```python
from build123d import *

# Parameters (mm, degrees)
Y_KSEKLIK_EKSTR_ZYON2_DEPTH       = 14
KES_EKSTR_ZYON1_REACH             = 47.202
IZIM2_R                           = 2.85
KES_EKSTR_ZYON1_DIRECTION_2_DEPTH = 46.202322949


with BuildPart() as part:
    # Çizim1 → Yükseklik-Ekstrüzyon2 (new body)
    with BuildSketch(Plane.XY):
        with BuildLine():
            Line((21, -23), (-21, -23))
            Line((-21, -23), (-21, -16.5))
            Line((-21, -16.5), (-10, -16.5))
            Line((-10, -16.5), (-10, 14.5))
            Line((-10, 14.5), (-0.5, 14.5))
            Line((-0.5, 14.5), (-0.5, 5.979130372))
            ThreePointArc((-0.5, 5.979130372), (0, -6), (0.5, 5.979130372))
            Line((0.5, 5.979130372), (0.5, 14.5))
            Line((0.5, 14.5), (10, 14.5))
            Line((10, 14.5), (10, -16.5))
            Line((10, -16.5), (21, -16.5))
            Line((21, -16.5), (21, -23))
        make_face()
    extrude(amount=Y_KSEKLIK_EKSTR_ZYON2_DEPTH)

    # Çizim2 → Kes-Ekstrüzyon1 (cut, up to next)
    with BuildSketch(Plane.XZ.offset(23), mode=Mode.PRIVATE) as kes_ekstr_zyon1_sk1:
        with Locations(Location((-16.05, 7, 0), (0, 0, 90))):
            Circle(IZIM2_R)
    kes_ekstr_zyon1_tool1 = extrude(kes_ekstr_zyon1_sk1.sketch, amount=-KES_EKSTR_ZYON1_REACH, mode=Mode.PRIVATE) & part.part
    # Çizim2 → Kes-Ekstrüzyon1 (cut, up to next)
    with BuildSketch(Plane.XZ.offset(23), mode=Mode.PRIVATE) as kes_ekstr_zyon1_sk2:
        with Locations(Location((16.05, 7, 0), (0, 0, 90))):
            Circle(IZIM2_R)
    kes_ekstr_zyon1_tool2 = extrude(kes_ekstr_zyon1_sk2.sketch, amount=-KES_EKSTR_ZYON1_REACH, mode=Mode.PRIVATE) & part.part
    add(kes_ekstr_zyon1_tool1.solids().sort_by_distance((-16.05, -23, 7))[0], mode=Mode.SUBTRACT)
    add(kes_ekstr_zyon1_tool2.solids().sort_by_distance((16.05, -23, 7))[0], mode=Mode.SUBTRACT)

    # Çizim2 → Kes-Ekstrüzyon1 direction 2 (cut)
    with BuildSketch(Plane.XZ.offset(23)):
        with Locations(Location((-16.05, 7, 0), (0, 0, 90))):
            Circle(IZIM2_R)
        with Locations(Location((16.05, 7, 0), (0, 0, 90))):
            Circle(IZIM2_R)
    extrude(amount=KES_EKSTR_ZYON1_DIRECTION_2_DEPTH, mode=Mode.SUBTRACT)


solid = part.part
```
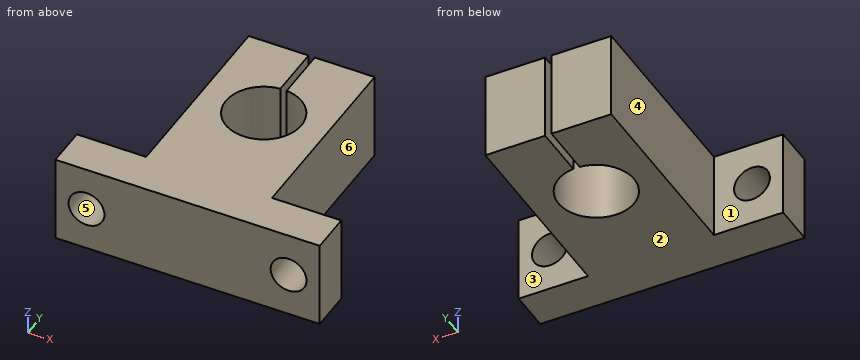
CAD build for the part. Positions are in the model's coordinates, mm. Face numbers are marked on the shaded views. A direction names the side the tool comes from. Round coordinates to 2 decimals unless told otherwise and drop trailing zeros. Order: outer loops, then holes, each group sorted by start corner. A loop starts at its lowest first (then second) coordinate and runs counter-clockwise, first axis right, second up.
Q1. Slice it at C-C (x = -16.05). Write the cut outline in (y, z), and give its area (4 significant figures).
Q2. Slice it at D-D (z = 12). Write the cut outline in (x, y).
Q3. Slice it at A-A (y = 0). Write the cut outline in (x, z).
Q4. Wall check: L1, parallel to X at y = -19.5, z = 7; L2, parallel to Z at x = -16, y = -21; L3, parallel to X at y = 0, z = 7.75. Give the ranges that are in metal, low to high.
Q5. Slice it at B-B (z = 7). Write the cut outline in (x, y), and give its area (3 significant figures).
Q6. Drop flat-ended pins along their axis: pin 1 (4.5 mm diameter, centred on y = 11.5, z = 3.5, fed in from -X); pin 2 (3.5 mm diameter, centred on x = -13, z = 6, fed in from +Y); pin 3 (4 mm diameter, centred on y = -4.5, z = 8, fed in from +X); pin 4 (3.5 mm diameter, centred on x = 16.05, z = 7, fed in from -Y). Give the stop position or say it passes through.
Q7. Which spindle directions (+Z, -Z, +X, -X, +Y, -Y) get a long thin tool onto all of the face, cutting with end or side? Do the marked faces 1, 2 and 3. Say none if no direction does.
Q8. Two-plate mould, pull along X, no slides. Class the marked faces 4, 5 and 6: pulls with the +X half, pulls with the -X half, needs draft (parallel to the pull), parting line crosses it, or undercut.
Results below:
1. outline: (-23, 0) - (-16.5, 0) - (-16.5, 4.15) - (-23, 4.15) - close; (-23, 9.85) - (-16.5, 9.85) - (-16.5, 14) - (-23, 14) - close
1. area: 53.95 mm2
2. outline: (-21, -23) - (21, -23) - (21, -16.5) - (10, -16.5) - (10, 14.5) - (0.5, 14.5) - (0.5, 5.98) arc R6 cw (long way) to (-0.5, 5.98) - (-0.5, 14.5) - (-10, 14.5) - (-10, -16.5) - (-21, -16.5) - close
3. outline: (-10, 0) - (-6, 0) - (-6, 14) - (-10, 14) - close; (6, 0) - (10, 0) - (10, 14) - (6, 14) - close
4. L1: x = -21 to -18.9, -13.2 to 13.2, 18.9 to 21
4. L2: z = 0 to 4.15, 9.85 to 14
4. L3: x = -10 to -6, 6 to 10
5. outline: (-21, -23) - (-18.9, -23) - (-18.9, -16.5) - (-21, -16.5) - close; (-13.2, -23) - (13.2, -23) - (13.2, -16.5) - (10, -16.5) - (10, 14.5) - (0.5, 14.5) - (0.5, 5.98) arc R6 cw (long way) to (-0.5, 5.98) - (-0.5, 14.5) - (-10, 14.5) - (-10, -16.5) - (-13.2, -16.5) - close; (18.9, -23) - (21, -23) - (21, -16.5) - (18.9, -16.5) - close
5. area: 697 mm2
6. pin 1: stops at x = -10
6. pin 2: stops at y = -16.5
6. pin 3: stops at x = 10
6. pin 4: passes through
7. face 1: +Z, -Z, -X, +Y
7. face 2: -Z, +X, -X, +Y, -Y
7. face 3: +Z, -Z, +X, +Y
8. face 4: pulls with the -X half
8. face 5: undercut
8. face 6: pulls with the +X half
